from build123d import *

# Parameters (mm, degrees)
F0_W     = 418
F0_H     = 568
F0_W_2   = 382.000006
F0_H_2   = 532.000006
F1_DEPTH = 69
F0_W_3   = 280
F0_H_3   = 430
F2_DEPTH = 18
F3_DEPTH = 3


with BuildPart() as f1:
    # F0 (on Top) → F1 (new body)
    with BuildSketch(Plane.XY):
        Rectangle(F0_W, F0_H)
        Rectangle(F0_W_2, F0_H_2, mode=Mode.SUBTRACT)
    extrude(amount=F1_DEPTH)

    # F0 (on Top) → F2 (join)
    with BuildSketch(Plane.XY):
        Rectangle(F0_W, F0_H)
        Rectangle(F0_W_2, F0_H_2, mode=Mode.SUBTRACT)
        Rectangle(F0_W_2, F0_H_2)
        Rectangle(F0_W_3, F0_H_3, mode=Mode.SUBTRACT)
    extrude(amount=F2_DEPTH)

    # F0 (on Top) → F3 (join)
    with BuildSketch(Plane.XY):
        Rectangle(F0_W_2, F0_H_2)
        Rectangle(F0_W_3, F0_H_3, mode=Mode.SUBTRACT)
        Rectangle(F0_W_3, F0_H_3)
    extrude(amount=F3_DEPTH)


solid = f1.part
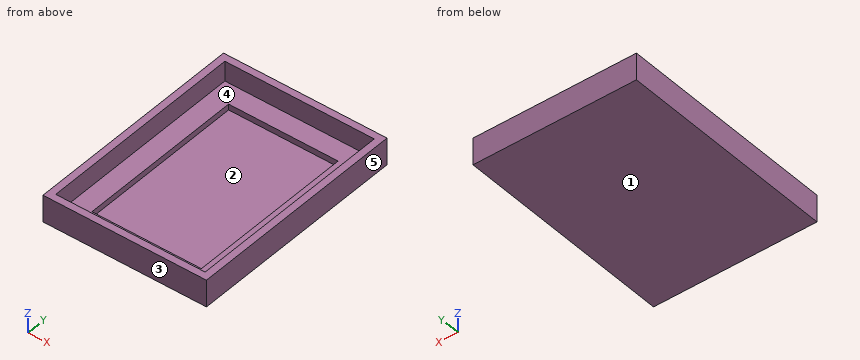
CAD build for the part. Positions are in the model's coordinates, mm. Face numbers are marked on the shaded views. A direction names the side the tool comes from. Give positions to 0.01 mm unless a question says otherwise; leave off trailing zeros. Loops run counter-clockwise (first coordinate to the right, second up) from the corner with the lowest first, then second, coordinate; pieces in that order, holes last. Notation, with made-up numbers: M 11.25,78 L 68.25,78 A10 cw 68.25,88 Z; hole C 89.5,59.25 d3. An arc over 180 degrees is marked long. Write each question's results on one line, items separated by ' | '.
Q1. Probe probe 1 along X at (y, z) = (130, 16); probe 2 along X at (y, z) = (108, 64); probe 3 along Y at (x, z) = (-66.5, 32). List the from-to ranges inside material, lowest first.
Geometry check:
probe 1: x = -209 to -140, 140 to 209 | probe 2: x = -209 to -191, 191 to 209 | probe 3: y = -284 to -266, 266 to 284
Q2. Flat gauge pins, fed straight in: P1, Ø5, axis at x = 138.5, y = -63, coming from the +Z side; P2, Ø6, axis at x = -74, y = 23, coming from the +Z side. Where does each tip first touch, or does it go through?
Geometry check:
P1: stops at z = 18 | P2: stops at z = 3
Q3. Band-saw the part on B-B on y = 204. Write the cut outline in (x, z).
Geometry check:
outline: M -209,0 L 209,0 L 209,69 L 191,69 L 191,18 L 140,18 L 140,3 L -140,3 L -140,18 L -191,18 L -191,69 L -209,69 Z
Q4. Band-saw the part on A-A on x = -78.5. Write the cut outline in (y, z), and give its area (3 significant figures).
Geometry check:
outline: M -284,0 L 284,0 L 284,69 L 266,69 L 266,18 L 215,18 L 215,3 L -215,3 L -215,18 L -266,18 L -266,69 L -284,69 Z | area: 5,610 mm²
Q5. Band-saw the part on C-C on z = 39.5. Write the cut outline in (x, y).
Geometry check:
outline: M -209,-284 L 209,-284 L 209,284 L -209,284 Z; hole M -191,-266 L 191,-266 L 191,266 L -191,266 Z
Q6. Which spindle directions (+Z, -Z, +X, -X, +Y, -Y) get a long thin tool onto all of the face, cutting with end or side? Do the marked faces 1 and 2. Say none if no direction does.
Geometry check:
face 1: -Z, +X, -X, +Y, -Y | face 2: +Z
Q7. Mould opens along Y. For the marked faces 3, 4 and 5 say: pulls with the +Y half, pulls with the -Y half, needs draft (parallel to the pull), parting line crosses it, or undercut.
Geometry check:
face 3: pulls with the -Y half | face 4: undercut | face 5: needs draft
